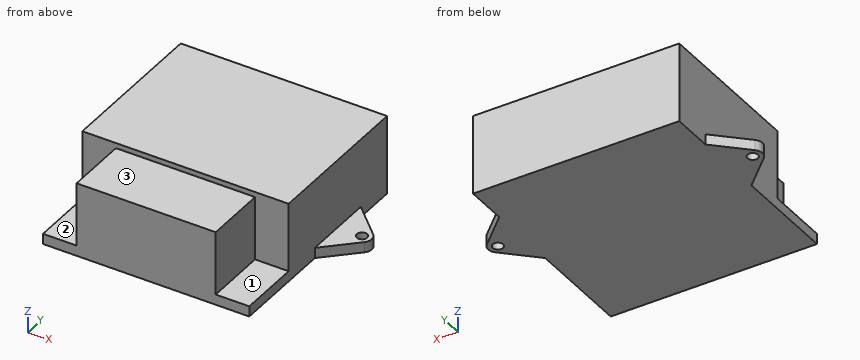
```python
from build123d import *

# Parameters (mm, degrees)
F1_DEPTH = 19.304
F0_W     = 33.8328
F0_H     = 15.24
F2_DEPTH = 18.034
F0_W_2   = 8.1661
F0_R     = 1.27
F3_DEPTH = 2.54


with BuildPart() as f1:
    # F0 (on Top) → F1 (new body)
    with BuildSketch(Plane.XY):
        Polygon((25.0825, 8.89), (25.0825, 19.05), (-25.0825, 19.05), (-25.0825, 8.89), (-25.0825, -8.89), (-25.0825, -19.05), (-16.9164, -19.05), (16.9164, -19.05), (25.0825, -19.05), (25.0825, -8.89), align=None)
    extrude(amount=F1_DEPTH)

    # F0 (on Top) → F2 (join, through all)
    with BuildSketch(Plane.XY):
        with Locations((0, -26.67)):
            Rectangle(F0_W, F0_H)
    extrude(amount=F2_DEPTH)

    # F0 (on Top) → F3 (join)
    with BuildSketch(Plane.XY):
        with Locations((-20.99945, -26.67)):
            Rectangle(F0_W_2, F0_H)
        with Locations((20.99945, -26.67)):
            Rectangle(F0_W_2, F0_H)
        with BuildLine():
            Line((-25.0825, -8.89), (-25.0825, 8.89))
            Line((-25.0825, 8.89), (-32.608938648, 1.7030678618))
            ThreePointArc((-32.608938648, 1.7030678618), (-33.3375, 0), (-32.608938648, -1.7030678618))
            Line((-32.608938648, -1.7030678618), (-25.0825, -8.89))
        make_face()
        with Locations((-30.9826936573, 0)):
            Circle(F0_R, mode=Mode.SUBTRACT)
        with BuildLine():
            Line((32.608938648, 1.7030678618), (25.0825, 8.89))
            Line((25.0825, 8.89), (25.0825, -8.89))
            Line((25.0825, -8.89), (32.608938648, -1.7030678618))
            ThreePointArc((32.608938648, -1.7030678618), (33.3375, 0), (32.608938648, 1.7030678618))
        make_face()
        with Locations((30.9826936573, 0)):
            Circle(F0_R, mode=Mode.SUBTRACT)
    extrude(amount=F3_DEPTH)


solid = f1.part
```
Design review of the part built by this model. Coordinates are the model's own, in mm. Face numbers are marked on the shaded views. A direction names the side the tool comes from. Coordinates: 2 decimals unless noted, no trailing zeros. Write each loop counter-clockwise with the first axis right and the second up, starting at its lowest first coordinate (ties: lowest second). Pieces come first, ordered by that corner, then holes.
1) Insertion check: pin 1 (8 mm diameter, centred on y = 9.5, z = 15, fed in from -X); pin 2 (4 mm diameter, centred on x = 22.5, y = -24.5, fed in from +Z); pin 3 (1 mm diameter, centred on y = -22, z = 6, fed in from +X). Each pin has a flat end and moves straight along its axis. Give the tip position at first contact, or say it passes through.
2) Add section A-A (y = 0). Write out the cut boundary in (x, z), plus the area to 3 significant figures.
3) Add section B-B (z = 8.75). Write out the cut boundary in (x, y).
4) Add section D-D (y = -17.5). Write out the cut boundary in (x, z).
5) To check wall thickness, follow L1, parallel to X at y = 1, z = 13.75; L2, parallel to Z at x = -11.5, y = -28; L3, parallel to Y at x = 22, z = 13. State the ranges of each line that lie inside material, in increasing order.
6) Machinability: for the marked faces 1, 2 and 3, which of the approach directions +Z, -Z, +X, -X, +Y, -Y give a long, thin tool a straight path to every point of the face, cutting with its end or side? Answer none if there is none.
7) Add section C-C (x = -15.5). Write out the cut boundary in (y, z), plus the area to 3 significant figures.
Check result:
1. pin 1: stops at x = -25.08
1. pin 2: stops at z = 2.54
1. pin 3: stops at x = 16.92
2. outline: (-33.34, 0) - (-32.25, 0) - (-32.25, 2.54) - (-33.34, 2.54) - close; (-29.71, 0) - (29.71, 0) - (29.71, 2.54) - (25.08, 2.54) - (25.08, 19.3) - (-25.08, 19.3) - (-25.08, 2.54) - (-29.71, 2.54) - close; (32.25, 0) - (33.34, 0) - (33.34, 2.54) - (32.25, 2.54) - close
2. area: 997 mm2
3. outline: (-25.08, -19.05) - (-16.92, -19.05) - (-16.92, -34.29) - (16.92, -34.29) - (16.92, -19.05) - (25.08, -19.05) - (25.08, 19.05) - (-25.08, 19.05) - close
4. outline: (-25.08, 0) - (25.08, 0) - (25.08, 19.3) - (-25.08, 19.3) - close
5. L1: x = -25.08 to 25.08
5. L2: z = 0 to 18.03
5. L3: y = -19.05 to 19.05
6. face 1: +Z, +X, -Y
6. face 2: +Z, -X, -Y
6. face 3: +Z, +X, -X, -Y
7. outline: (-34.29, 0) - (19.05, 0) - (19.05, 19.3) - (-19.05, 19.3) - (-19.05, 18.03) - (-34.29, 18.03) - close
7. area: 1,010 mm2
